Here's how the part is built. I have some questions about the finished solid (model axes, mm). Face numbers are marked on the shaded views. Coordinates: 2 decimals unless noted, no trailing zeros. Loops run counter-clockwise (first coordinate to the right, second up) from the corner with the lowest first, then second, coordinate; pieces in that order, holes last.
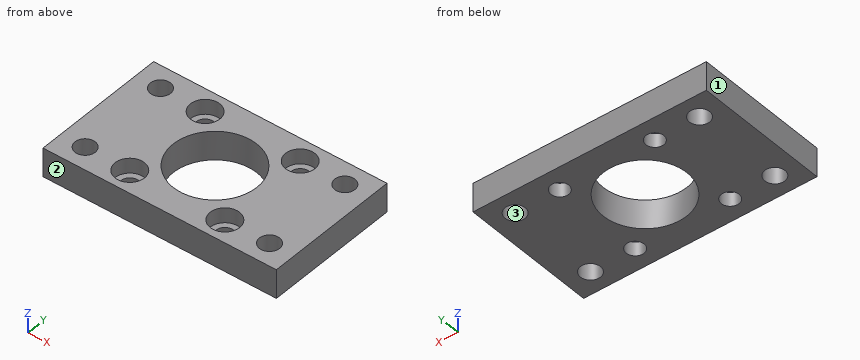
from build123d import *

# Parameters (mm, degrees)
ESQUISSE2_W             = 81
ESQUISSE2_H             = 47
ESQUISSE2_R             = 14.5
ESQUISSE2_R_2           = 3.5
ESQUISSE2_R_3           = 3.1
BOSS_EXTRU_1_DEPTH      = 10
ESQUISSE5_R             = 5.1
ENL_V_MAT_EXTRU_1_DEPTH = 5.2


with BuildPart() as part:
    # Esquisse2 → Boss.-Extru.1 (new body)
    with BuildSketch(Plane.XY):
        with Locations((40.5, 23.5)):
            Rectangle(ESQUISSE2_W, ESQUISSE2_H)
        with Locations((40.5, 23.5)):
            Circle(ESQUISSE2_R, mode=Mode.SUBTRACT)
        with Locations((8.5, 39.5)):
            Circle(ESQUISSE2_R_2, mode=Mode.SUBTRACT)
        with Locations((72.5, 39.5)):
            Circle(ESQUISSE2_R_2, mode=Mode.SUBTRACT)
        with Locations((72.5, 7.5)):
            Circle(ESQUISSE2_R_2, mode=Mode.SUBTRACT)
        with Locations((8.5, 7.5)):
            Circle(ESQUISSE2_R_2, mode=Mode.SUBTRACT)
        with Locations((24, 39.5)):
            Circle(ESQUISSE2_R_3, mode=Mode.SUBTRACT)
        with Locations(Location((57, 39.5, 0), (0, 0, 180))):  # turned: the seam where the file's is
            Circle(ESQUISSE2_R_3, mode=Mode.SUBTRACT)
        with Locations((57, 7.5)):
            Circle(ESQUISSE2_R_3, mode=Mode.SUBTRACT)
        with Locations(Location((24, 7.5, 0), (0, 0, 180))):  # turned: the seam where the file's is
            Circle(ESQUISSE2_R_3, mode=Mode.SUBTRACT)
    extrude(amount=BOSS_EXTRU_1_DEPTH)

    # Esquisse5 → Enlèv. mat.-Extru.1 (cut)
    with BuildSketch(Plane.XY.offset(10)):
        with Locations((24, 39.5)):
            Circle(ESQUISSE5_R)
        with Locations((24, 7.5)):
            Circle(ESQUISSE5_R)
        with Locations((57, 7.5)):
            Circle(ESQUISSE5_R)
        with Locations((57, 39.5)):
            Circle(ESQUISSE5_R)
    extrude(amount=-ENL_V_MAT_EXTRU_1_DEPTH, mode=Mode.SUBTRACT)


solid = part.part
Q1. Please list where these lines run through material, in increasing order: probe 1 along Y at (x, z) = (57, 6.05); probe 2 along Y at (x, z) = (57, 1.6); probe 3 along Y at (x, z) = (40.5, 6).
Q2. Suppose I cut it at C-C on z = 1.75. State how many separate pieces and enclosed holes the cut face has, and give its area (3 significant figures).
Q3. Suppose I cut it at D-D on y = 23.5. Write out the boundary of the cut face in (x, z).
Q4. Suppose I cut it at A-A on y = 7.5. Write out the boundary of the cut face in (x, z), and give its area (3 significant figures).
Q5. We'd pull the mould along X, two halves only. Please class the marked faces 1, 2 and 3: pulls with the +X half, pulls with the -X half, needs draft (parallel to the pull), parting line crosses it, or undercut.
Q6. Suppose I cut it at B-B on x = 8.5. Write out the boundary of the cut face in (y, z).
Q7. Will these pins go through, and if not, where does the flat tip stop? P1, Ø4, axis at x = 72.5, y = 39.5, coming from the +Z side; P2, Ø5, axis at x = 58.5, y = 5.5, coming from the +Z side.
Check values:
1. probe 1: y = 0 to 2.4, 12.6 to 34.4, 44.6 to 47
1. probe 2: y = 0 to 4.4, 10.6 to 36.4, 42.6 to 47
1. probe 3: y = 0 to 9, 38 to 47
2. separate pieces: 1
2. enclosed holes: 9
2. area: 2,870 mm2
3. outline: (0, 0) - (26, 0) - (26, 10) - (0, 10) - close; (55, 0) - (81, 0) - (81, 10) - (55, 10) - close
4. outline: (0, 0) - (5, 0) - (5, 10) - (0, 10) - close; (12, 0) - (20.9, 0) - (20.9, 4.8) - (18.9, 4.8) - (18.9, 10) - (12, 10) - close; (27.1, 0) - (53.9, 0) - (53.9, 4.8) - (51.9, 4.8) - (51.9, 10) - (29.1, 10) - (29.1, 4.8) - (27.1, 4.8) - close; (60.1, 0) - (69, 0) - (69, 10) - (62.1, 10) - (62.1, 4.8) - (60.1, 4.8) - close; (76, 0) - (81, 0) - (81, 10) - (76, 10) - close
4. area: 504 mm2
5. face 1: pulls with the -X half
5. face 2: needs draft
5. face 3: undercut
6. outline: (0, 0) - (4, 0) - (4, 10) - (0, 10) - close; (11, 0) - (36, 0) - (36, 10) - (11, 10) - close; (43, 0) - (47, 0) - (47, 10) - (43, 10) - close
7. P1: passes through
7. P2: stops at z = 4.8
